Check sheet for the drawn part. Datum: minimum x, y, z corner. Units: mm. A direction names the side the tool comes from. Round coordinates to 2 decimals unless told otherwise and drop trailing zeros. Write each loop counter-clockwise with the first axis right and the second up, starting at its lowest first coordinate (ties: lowest second). Pieces come first, ordered by that corner, then holes. Notation, with made-up numbers: M 53.5,29 L 103.5,29 A33 ccw 103.5,59 Z; hole C 23,38 d7. An arc over 180 degrees is marked long. Answer in a Markdown table with one row per item. Add a question column.
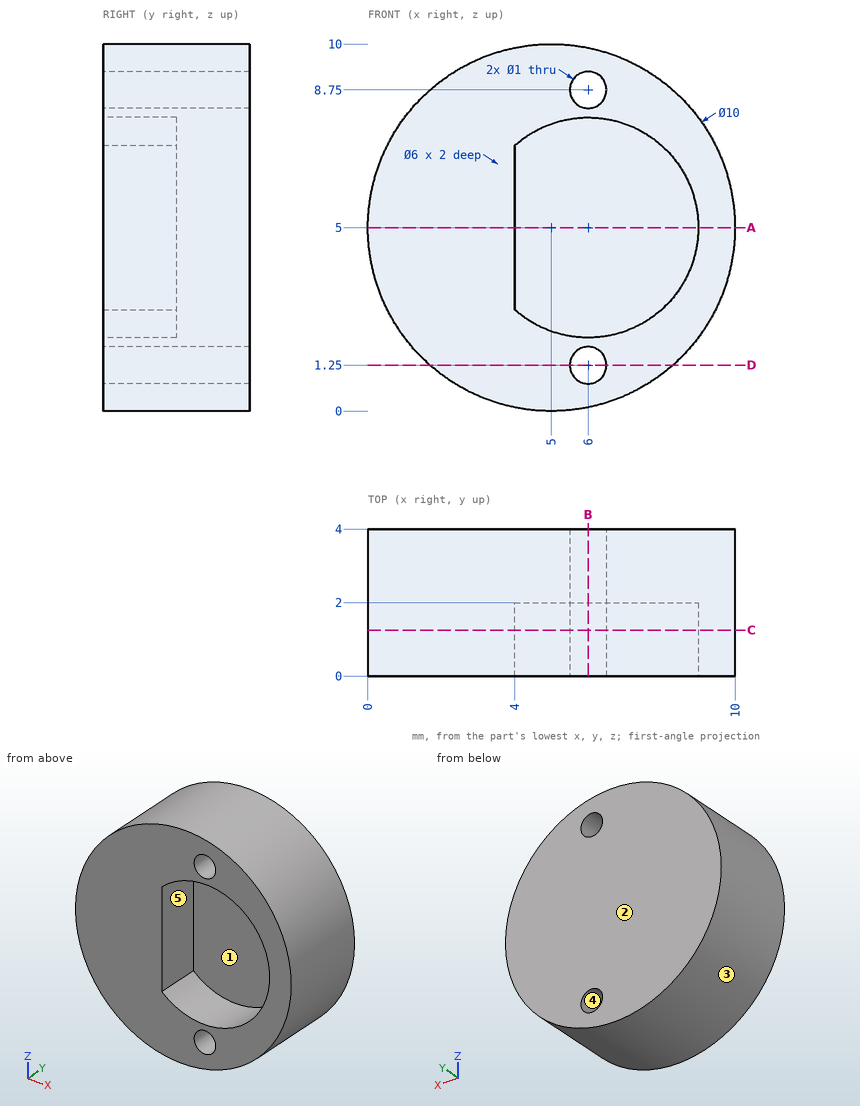
Item 1: Section check A-A, the plane z = 5. Record the boundary of the cut face in (x, y).
Item 2: Access from +Z, -Z, +X, -X, +Y, -Y to the whole of each face (thin tool, end or side, straight path). Record for the marked faces 4 and 5.
Item 3: Section check D-D, the plane z = 1.25. Record the boundary of the cut face in (x, y).
Item 4: Gauge pin test, flat ends, axial feed: pin 1 Ø1.5 at (y, z) = (2.5, 8) entering from -X; pin 2 Ø0.6 at (y, z) = (0.5, 5.5) entering from +X; pin 3 Ø2 at (x, z) = (4.5, 7) entering from -Y; pin 4 Ø1.5 at (x, z) = (6.5, 5) entering from -Y. Record the tip position at first contact, or that the pin passes through.
Item 5: Section check C-C, the plane y = 1.25. Record the boundary of the cut face in (x, z), and give its area (3 significant figures).
Item 6: Section check B-B, the plane x = 6. Record the boundary of the cut face in (y, z).
Item 7: Mould release check, pull along X, two halves, no side actions. Record for the marked faces 1, 2 and 3: +X half, -X half, draft (parallel to the pull), parting line (faces both ways), or undercut.
Item 8: Scan lines: probe 1 along Z at (x, y) = (6, 1.05); probe 2 along Y at (x, z) = (7.75, 7.25); probe 3 along X at (y, z) = (0.35, 5). Record each from-to range of solid material in increasing order. Write a range as from..to.
Result sheet:
| question | item | result |
|---|---|---|
| 1 | outline | M 0,0 L 4,0 L 4,2 L 9,2 L 9,0 L 10,0 L 10,4 L 0,4 Z |
| 2 | face 4 | +Y, -Y |
| 2 | face 5 | -Y |
| 3 | outline | M 1.69,0 L 5.5,0 L 5.5,4 L 1.69,4 Z; M 6.5,0 L 8.31,0 L 8.31,4 L 6.5,4 Z |
| 4 | pin 1 | stops at x = 0.53 |
| 4 | pin 2 | stops at x = 10 |
| 4 | pin 3 | stops at y = 0 |
| 4 | pin 4 | stops at y = 2 |
| 5 | outline | C 5,5 d10; hole M 4,2.76 A3 ccw long 4,7.24 Z; hole C 6,1.25 d1; hole C 6,8.75 d1 |
| 5 | area | 51.8 mm^2 |
| 6 | outline | M 0,0.1 L 4,0.1 L 4,0.75 L 0,0.75 Z; M 0,1.75 L 4,1.75 L 4,8.25 L 0,8.25 L 0,8 L 2,8 L 2,2 L 0,2 Z; M 0,9.25 L 4,9.25 L 4,9.9 L 0,9.9 Z |
| 7 | face 1 | undercut |
| 7 | face 2 | draft |
| 7 | face 3 | parting line |
| 8 | probe 1 | z = 0.1..0.75, 1.75..2, 8..8.25, 9.25..9.9 |
| 8 | probe 2 | y = 2..4 |
| 8 | probe 3 | x = 0..4, 9..10 |
